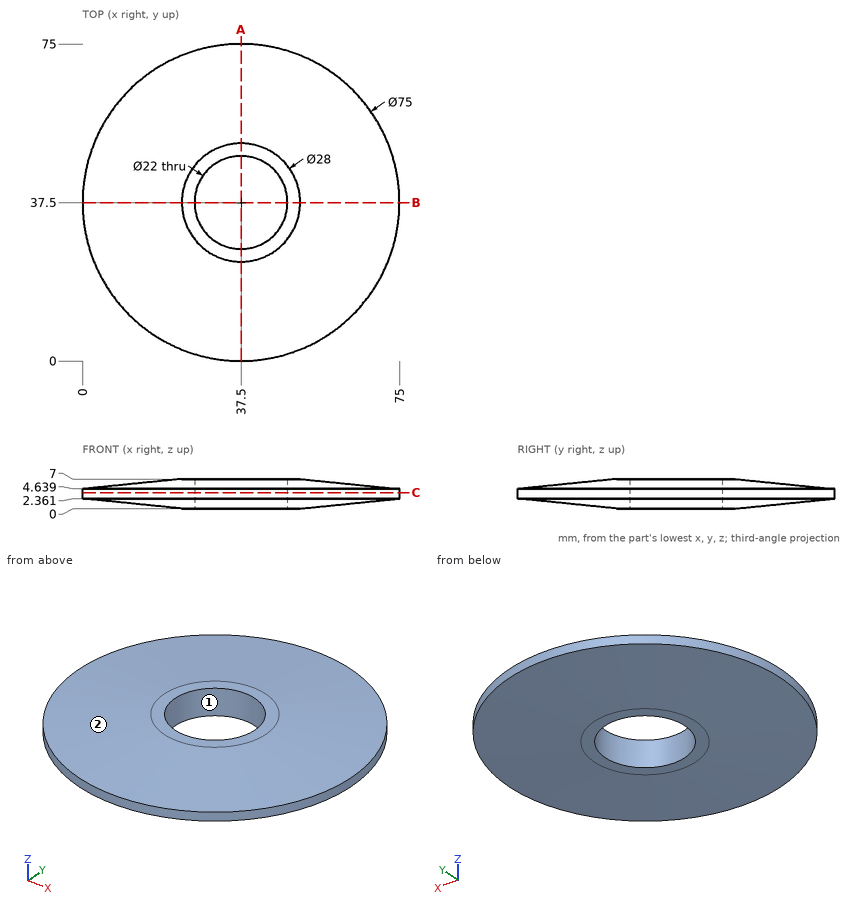
Part print with two shaded views. Sizes in mm from the minimum x, y, z corner. Coordinates: 2 decimals unless noted, no trailing zeros. Write each loop counter-clockwise with the first axis right and the second up, starting at its lowest first coordinate (ties: lowest second). Pieces come first, ordered by that corner, then holes. Notation, with made-up numbers: (-22, -3.5) -> (-10, -3.5) arc R37 ccw to (-10, 34.5) -> close; hole circle Ø8 at (73.25, 81.25). An arc over 180 degrees is marked (long way). Return JSON: item names as keys, results as strings. Group by question number.
Q1. Flat gauge pins, fed straight in: pin 1 (1.5 mm diameter, centred on x = 20, y = 66.5, fed in from -Z); pin 2 (3 mm diameter, centred on x = 11, y = 28, fed in from +Z); pin 3 (4 mm diameter, centred on x = 21, y = 52.5, fed in from +Z). Where does each tip first touch, or does it go through?
Q2. Cut at C-C, the plane z = 3.75. Give the cut face in (x, y).
Q3. Cut at A-A, the plane x = 37.5. Give the cut face in (y, z), then the cut area to 3 significant figures.
Q4. Drill centre lines: line 1 (Y direction, x = 37.5, z = 3.5); line 2 (Y direction, x = 34, z = 4.5); line 3 (Z direction, x = 20, y = 70.5). Where is each one in solid material? Low to high.
Q5. Pull direction Y, two halves, no side cores. Call the marked faces 1 and 2: released by +Y, released by -Y, zero draft, split by the parting line, or undercut.
Returned:
{
 "1": {"pin 1": "stops at z = 1.92", "pin 2": "stops at z = 5.73", "pin 3": "stops at z = 6.37"},
 "2": {"outline": "circle Ø75 at (37.5, 37.5); hole circle Ø22 at (37.5, 37.5)"},
 "3": {"outline": "(0, 2.36) -> (23.5, 0) -> (26.5, 0) -> (26.5, 7) -> (23.5, 7) -> (0, 4.64) -> close; (48.5, 0) -> (51.5, 0) -> (75, 2.36) -> (75, 4.64) -> (51.5, 7) -> (48.5, 7) -> close", "area": "260 mm2"},
 "4": {"line 1": "y = 0 to 26.5, 48.5 to 75", "line 2": "y = 0.16 to 27.07, 47.93 to 74.84", "line 3": "z = 2.35 to 4.65"},
 "5": {"face 1": "undercut", "face 2": "split by the parting line"}
}
